```python
from build123d import *

# Parameters (mm, degrees)
F0_W     = 10.16
F0_H     = 10.16
F1_DEPTH = 6.35
F2_R     = 0.889
F3_DEPTH = 25.4
F5_DEPTH = 6.35


with BuildPart() as f1:
    # F0 (on Front) → F1 (new body)
    with BuildSketch(Plane.XZ):
        Rectangle(F0_W, F0_H)
    extrude(amount=F1_DEPTH)

    # F2 (on face) → F3 (cut)
    with BuildSketch(Plane.YZ.offset(5.08)):
        with Locations((-3.175, 0)):
            Circle(F2_R)
    extrude(amount=-F3_DEPTH, mode=Mode.SUBTRACT)

    # F4 (on Front) → F5 (join)
    with BuildSketch(Plane.XZ):
        with BuildLine():
            ThreePointArc((-14.516378, -10.212987), (-14.12825, -14.686308), (-9.654929, -14.298181))
            ThreePointArc((-9.654929, -14.298181), (-4.445, 0), (-9.654929, 14.298181))
            ThreePointArc((-9.654929, 14.298181), (-14.12825, 14.686308), (-14.516378, 10.212987))
            ThreePointArc((-14.516378, 10.212987), (-10.795, 0), (-14.516378, -10.212987))
        make_face()
        with BuildLine():
            ThreePointArc((-10.841122, 13.301393), (-5.9944, 0), (-10.841122, -13.301393))
            ThreePointArc((-10.841122, -13.301393), (-13.131463, -13.500114), (-13.330184, -11.209774))
            ThreePointArc((-13.330184, -11.209774), (-9.2456, 0), (-13.330184, 11.209774))
            ThreePointArc((-13.330184, 11.209774), (-13.131463, 13.500114), (-10.841122, 13.301393))
        make_face(mode=Mode.SUBTRACT)
    extrude(amount=F5_DEPTH)


solid = f1.part
```
Source: CAD feature listing. Evaluate the final solid. Frame: model axes, mm. A direction names the side the tool comes from. Give positions to 0.01 mm unless a question says otherwise; leave off trailing zeros. Order: outer loops, then holes, each group sorted by start corner. A loop starts at its lowest first (then second) coordinate and runs counter-clockwise, first axis right, second up.
(1) Material intervals for line 1 along Y through (x, z) = (-1.25, 0); line 2 along Z through (x, y) = (-10.75, -4.25); line 3 along X through (y, z) = (-4.75, 0) (3 decimals), sorted ascending.
(2) Section query B-B (y = -0.5). Return the cut outline in (x, z) (3 decimals), plus the area to 3 significant figures.
(3) Pull-direction query (X, two-part tool) for faces 1 (the face through (0, -3, -5.08)), 2 (the face through (-13.159, -3.131, 13.477)), 3 (the face through (-14.074, -3.131, 14.731)); classes: +X half, -X half, draft (parallel to the pull), parting line (faces both ways), or undercut.
(4) Contact query for flat-ended pins moving along their axis: P1, Ø3, axis at x = -1.5, y = -3, coming from the -Z side; P2, Ø3, axis at y = -3.175, z = 0, coming from the -X side. Output: stop coordinate, or through.
(5) Section query A-A (z = -8). Return the cut outline in (x, y), plus the area to 3 significant figures.
(6) Access query for faces 4 (the face through (5.08, -3.1, 1.1)), 5 (the face through (-6.835, -3.131, -10.026)), 6 (the face through (0.375, -4.063, 0.039)), 7 (the face through (0, -3, 5.08)), 8 (the face through (-9.246, -3.131, -0.17)). Directions: +Z, -Z, +X, -X, +Y, -Y. A direction counts if a zero-diameter tool reaches every point of the face in a straight line with its end or side. Return the directions, or none.
(7) Section query D-D (x = 1.25). Return the cut outline in (y, z) (3 decimals), plus the area to 3 significant figures.
(8) Section query C-C (x = -11.5). Return the cut outline in (y, z), plus the area to 3 significant figures.
Outcome:
1. line 1: y = -6.35 to -4.06, -2.29 to 0
1. line 2: z = -15.14 to -13.19, -7.08 to 7.08, 13.19 to 15.14
1. line 3: x = -10.795 to -9.246, -5.994 to 5.08
2. outline: (-14.516, -10.213) arc R3.175 ccw to (-9.655, -14.298) arc R22.225 ccw to (-5.033, -5.08) - (5.08, -5.08) - (5.08, 5.08) - (-5.033, 5.08) arc R22.225 ccw to (-9.655, 14.298) arc R3.175 ccw to (-14.516, 10.213) arc R15.875 cw to start; hole (-13.33, -11.21) arc R1.626 ccw to (-10.841, -13.301) arc R20.676 ccw to (-10.841, 13.301) arc R1.626 ccw to (-13.33, 11.21) arc R17.424 cw to start
2. area: 205 mm2
3. face 1: draft
3. face 2: undercut
3. face 3: parting line
4. P1: stops at z = -5.08
4. P2: stops at x = -10.87
5. outline: (-12.96, -6.35) - (-11.19, -6.35) - (-11.19, 0) - (-12.96, 0) - close; (-7.6, -6.35) - (-5.93, -6.35) - (-5.93, 0) - (-7.6, 0) - close
5. area: 21.8 mm2
6. face 4: +Z, -Z, +X, +Y, -Y
6. face 5: -Z, +X, +Y, -Y
6. face 6: +X
6. face 7: +Z, +X, +Y, -Y
6. face 8: +Y, -Y
7. outline: (-6.35, -5.08) - (0, -5.08) - (0, 5.08) - (-6.35, 5.08) - close; hole circle Ø1.778 at (-3.175, 0)
7. area: 62.0 mm2
8. outline: (-6.35, -15.38) - (0, -15.38) - (0, -13.77) - (-6.35, -13.77) - close; (-6.35, -8.57) - (0, -8.57) - (0, -4.68) - (-6.35, -4.68) - close; (-6.35, 4.68) - (0, 4.68) - (0, 8.57) - (-6.35, 8.57) - close; (-6.35, 13.77) - (0, 13.77) - (0, 15.38) - (-6.35, 15.38) - close
8. area: 69.8 mm2
